Read the model definition and answer for the solid it produces. Units are mm, in the model's axes. A direction names the side the tool comes from. Round coordinates to 2 decimals unless told otherwise and drop trailing zeros. Loops run counter-clockwise (first coordinate to the right, second up) from the corner with the lowest first, then second, coordinate; pieces in that order, holes last. Notation, with made-up numbers: M -16.5,-38 L 4.5,-38 A18 ccw 4.5,-16 Z; hole C 62.5,-10 d7. An arc over 180 degrees is marked long. Write each question's results on one line, items separated by ' | '.
Autodesk Inventor part; units mm, degrees
ref_plane "YZ Plane" through (0, 0, 0) normal (1, 0, 0) x (0, 1, 0)
ref_plane "XZ Plane" through (0, 0, 0) normal (0, 1, 0) x (-1, 0, 0)
ref_plane "XY Plane" through (0, 0, 0) normal (0, 0, 1) x (1, 0, 0)
sketch "Sketch1" plane through (0, 0, 0) normal (0, 1, 0) x (-1, 0, 0)
  line L0 (0, 0) -> (0, -25.4)
  line L1 (0, -25.4) -> (31.75, -25.4)
  line L2 (31.75, -25.4) -> (31.75, -10.668)
  line L3 (31.75, -10.668) -> (50.8, -10.668)
  line L4 (50.8, -10.668) -> (50.8, 10.668)
  line L5 (50.8, 10.668) -> (31.75, 10.668)
  line L6 (31.75, 10.668) -> (31.75, 25.4)
  line L7 (31.75, 25.4) -> (0, 25.4)
  line L8 (0, 25.4) -> (0, 0)
  line L9 (0, 0) -> (11.1125, 0)
  circle A0 centre (11.1125, 0) radius 11.1125
  dimension "d0" = 25.4
  dimension "d1" = 31.75
  dimension "d2" = 14.732
  dimension "d3" = 19.05
  dimension "d4" = 21.336
  dimension "d5" = 19.05
  dimension "d6" = 14.732
  dimension "d8" = 11.1125
extrude "Extrusion1" add sketch "Sketch1" along normal blind 1.27
equation "\"d5\" = d3"
equation "\"d6\" = d2"
properties part number "Base"
1. Which of the six approach directions +Z, -Z, +X, -X, +Y, -Y give full straight-line access (tool end or side, diameter ignored) to faces 1 (the face through (-41, 1, 10.668)), 2 (the face through (-25, 0, 0)), 3 (the face through (-41, 1, -10.668))?
Completed:
face 1: +Z, -X, +Y, -Y | face 2: +Z, -Z, +X, -X, -Y | face 3: -Z, -X, +Y, -Y
2. Find section D-D, the plane z = 14. Give the vertices of the cut face in (x, y).
Completed:
outline: M -31.75,0 L 0,0 L 0,1.27 L -31.75,1.27 Z
3. Find section A-A, the plane x = -15. Give the vertices of the cut face in (y, z), then the cut area to 3 significant figures.
Completed:
outline: M 0,-25.4 L 1.27,-25.4 L 1.27,-10.41 L 0,-10.41 Z; M 0,10.41 L 1.27,10.41 L 1.27,25.4 L 0,25.4 Z | area: 38.1 mm2
4. Given P1, Ø0.6, axis at x = -41, y = 0.5, coming from the -Z side, flat-ended and moving along its own axis, determine where the tip first touches the part or whether it passes through.
Completed:
P1: stops at z = -10.67
5. Find the intervals of material crossed by L1, parallel to X at y = 0.25, z = -20.5; L2, parallel to Z at x = -36.5, y = 0.4; L3, parallel to X at y = 0.1, z = 4.5, in increasing order.
Completed:
L1: x = -31.75 to 0 | L2: z = -10.67 to 10.67 | L3: x = -50.8 to -21.27, -0.95 to 0
6. Find section B-B, the plane z = 2.5. Give the vertices of the cut face in (x, y), then the cut area to 3 significant figures.
Completed:
outline: M -50.8,0 L -21.94,0 L -21.94,1.27 L -50.8,1.27 Z; M -0.28,0 L 0,0 L 0,1.27 L -0.28,1.27 Z | area: 37.0 mm2
